Check sheet for the modelled part. Datum: model origin and axes. Units: mm. A direction names the side the tool comes from. Give positions to 0.01 mm unless a question says otherwise; leave off trailing zeros. Write each loop counter-clockwise with the first axis right and the second up, starting at its lowest first coordinate (ties: lowest second). Pieces come first, ordered by that corner, then holes. Notation, with made-up numbers: M 20.25,-32 L 75.25,-32 A29 cw 75.25,4 Z; hole C 12,14.5 d4. An arc over 180 degrees is marked long. Write item = value, one per line. Start each with the question number.
1) Cross-section at D-D, the plane x = -22.5. Record the cut outline in (y, z), plus the area to 3 significant figures.
2) Mould release check, pull along X, two halves, no side actions. Record for faces 4 (the flat face through (-25.4, 27, -6)), 5 (the flat face through (-13, -10.54, -25)), 6 (the flat face through (0, 19, -20)): released by +X, released by -X, zero draft, split by the parting line, or undercut.
3) Scan lines: line 1 along X through (y, z) = (37.5, -15.5); line 2 along Y through (x, z) = (-52.5, -27.5); line 3 along Y through (x, z) = (-21, 11). Record each from-to range of solid material in increasing order. Write a range as [from, to].
4) Cross-section at B-B, the plane z = -29.5. Record the cut outline in (x, y), plus the area to 3 significant figures.
5) Access from +Z, -Z, +X, -X, +Y, -Y to the whole of each face (thin tool, end or side, straight path). Record for faces 1 (the flat face through (-25.4, -23, -25)), 2 (the flat face through (-64, -10.54, -19)), 3 (the flat face through (-64, -23, -5.922)).
6) Cross-section at C-C, the plane y = 31. Record the cut outline in (x, z), plus the area to 3 significant figures.
7) Go/stop test with flat-tipped pins: pin 1 (3 mm diameter, centred on x = -42.5, y = 8, fed in from +Z); pin 2 (7.5 mm diameter, centred on x = -16, z = 4, fed in from -Y); pin 3 (20.5 mm diameter, centred on x = -8, y = -18, fed in from +Z). Record where each tip stops, or that it passes through.
8) Cross-section at A-A, the plane z = -8. Record the cut outline in (x, y).
```python
from build123d import *

# Parameters (mm, degrees)
F0_W      = 76.2
F0_H      = 12.7
F1_DEPTH  = 76.2
F2_W      = 25.4
F2_H      = 25.4
F3_DEPTH  = 12.7
F3_FACE_W = 25.4
F3_FACE_H = 25.4
F4_DEPTH  = 12.7
F5_DEPTH  = 38.1
F6_DEPTH  = 25.4


with BuildPart() as f1:
    # F0 (on Right) → F1 (new body)
    with BuildSketch(Plane.YZ):
        with Locations((2.160154, -37.671763)):
            Rectangle(F0_W, F0_H)
    extrude(amount=-F1_DEPTH)

    # F2 (on face) → F3 (join)
    with BuildSketch(Plane.XY.offset(-31.321763)):
        with Locations((-12.7, -23.239846)):
            Rectangle(F2_W, F2_H)
        with Locations((-63.5, -23.239846)):
            Rectangle(F2_W, F2_H)
        with Locations((-12.7, 27.560154)):
            Rectangle(F2_W, F2_H)
        with Locations((-63.5, 27.560154)):
            Rectangle(F2_W, F2_H)
    extrude(amount=F3_DEPTH)

    # F3_face (on face) → F4 (join)
    with BuildSketch(Plane(origin=(-63.5, -23.239846, -18.621763), x_dir=(1, 0, 0), z_dir=(0, 0, 1))):
        Rectangle(F3_FACE_W, F3_FACE_H)
    extrude(amount=F4_DEPTH)

    # F3_face (on face) → F5 (join)
    with BuildSketch(Plane(origin=(-63.5, -23.239846, -18.621763), x_dir=(1, 0, 0), z_dir=(0, 0, 1))):
        with Locations((50.8, 50.8)):
            Rectangle(F3_FACE_W, F3_FACE_H)
    extrude(amount=F5_DEPTH)

    # F3_face (on face) → F6 (join)
    with BuildSketch(Plane(origin=(-63.5, -23.239846, -18.621763), x_dir=(1, 0, 0), z_dir=(0, 0, 1))):
        with Locations((0, 50.8)):
            Rectangle(F3_FACE_W, F3_FACE_H)
    extrude(amount=F6_DEPTH)


solid = f1.part
```
Reply:
q1.outline = M -35.94,-44.02 L 40.26,-44.02 L 40.26,19.48 L 14.86,19.48 L 14.86,-31.32 L -10.54,-31.32 L -10.54,-18.62 L -35.94,-18.62 Z
q1.area = 2,580 mm2
q2.face_4 = undercut
q2.face_5 = zero draft
q2.face_6 = released by +X
q3.line_1 = [-76.2, -50.8], [-25.4, 0]
q3.line_2 = [-35.94, -10.54], [14.86, 40.26]
q3.line_3 = [14.86, 40.26]
q4.outline = M -76.2,-35.94 L -50.8,-35.94 L -50.8,-10.54 L -76.2,-10.54 Z; M -76.2,14.86 L -50.8,14.86 L -50.8,40.26 L -76.2,40.26 Z; M -25.4,-35.94 L 0,-35.94 L 0,-10.54 L -25.4,-10.54 Z; M -25.4,14.86 L 0,14.86 L 0,40.26 L -25.4,40.26 Z
q4.area = 2,580 mm2
q5.face_1 = +Z, +Y, -Y
q5.face_2 = +Z, +X, -X
q5.face_3 = +Z, +X, -X, -Y
q6.outline = M -76.2,-44.02 L 0,-44.02 L 0,19.48 L -25.4,19.48 L -25.4,-31.32 L -50.8,-31.32 L -50.8,6.78 L -76.2,6.78 Z
q6.area = 3,230 mm2
q7.pin_1 = -31.32
q7.pin_2 = 14.86
q7.pin_3 = -18.62
q8.outline = M -76.2,-35.94 L -50.8,-35.94 L -50.8,-10.54 L -76.2,-10.54 Z; M -76.2,14.86 L -50.8,14.86 L -50.8,40.26 L -76.2,40.26 Z; M -25.4,14.86 L 0,14.86 L 0,40.26 L -25.4,40.26 Z
